Autodesk Inventor part; units mm, degrees
ref_plane "YZ Plane" through (0, 0, 0) normal (1, 0, 0) x (0, 1, 0)
ref_plane "XZ Plane" through (0, 0, 0) normal (0, 1, 0) x (-1, 0, 0)
ref_plane "XY Plane" through (0, 0, 0) normal (0, 0, 1) x (1, 0, 0)
sketch "Sketch1" plane through (0, 0, 0) normal (0, 0, 1) x (1, 0, 0)
  line L0 (0, 0) -> (25.4, 0)
  line L1 (25.4, 0) -> (25.4, 520.7)
  line L2 (25.4, 520.7) -> (0, 520.7)
  line L3 (0, 520.7) -> (0, 0)
  dimension "d0" = 25.4
  dimension "d1" = 520.7
extrude "Extrusion1" add sketch "Sketch1" along normal blind 25.4
shell "Shell1" thickness 3.175 removed faces 2 at (16.9333, 520.7, 8.4667) at (8.4667, 0, 8.4667)
sketch "Sketch2" plane through (0, 0, 0) normal (0, 0, -1) x (-1, 0, 0)
  line L0 (0, 520.7) -> (0, 0)
  line L1 (-25.4, 520.7) -> (0, 520.7)
  circle A0 centre (-12.7, 495.3) radius 3.175
  dimension "d5" = 12.7
  dimension "d6" = 25.4
  dimension "d7" = 6.35
extrude "Extrusion2" cut sketch "Sketch2" against normal through all
properties part number "CentralColumnInner" material "Aluminum-6061"
Read the model definition and answer for the solid it produces. Units are mm, in the model's axes. A direction names the side the tool comes from. Round coordinates to 2 decimals unless told otherwise and drop trailing zeros. Order: outer loops, then holes, each group sorted by start corner. A loop starts at its lowest first (then second) coordinate and runs counter-clockwise, first axis right, second up.
1) The part is cut by section A-A on z = 8.5. Write down the section's boundary in (x, y) (3 decimals), plus the area to 3 significant figures.
2) A flat-ended cylindrical pin translates along its axis: pin 1 (4 mm diameter, centred on x = 12.7, y = 495.3, fed in from +Z). Find the tip coordinate at first contact, or state that the pin passes through.
3) The part is cut by section B-B on y = 78. Write down the section's boundary in (x, z) (3 decimals).
4) The mould has two halves that part along Z. Classify faces 3 (the face through (13, 264, 0)), 4 (the face through (13, 264, 25.4)), 5 (the face through (13, 264, 3.175)), 6 (the face through (25.4, 257, 13)): released by +Z, released by -Z, zero draft, split by the parting line, or undercut.
5) Straight lines are drawn through the part: L1, parallel to X at y = 495.3, z = 24.75 (3 decimals); L2, parallel to Z at x = 4.5, y = 63 (3 decimals). For each, find the intervals that lie inside material, in ascending order.
6) For faces 1 (the face through (2, 520.7, 13)), 2 (the face through (13, 264, 22.225)), determine the directions among +Z, -Z, +X, -X, +Y, -Y from which every point of the face is accessible in a straight line to the end or side of a thin tool.
Resolved:
1. outline: (0, 0) - (3.175, 0) - (3.175, 520.7) - (0, 520.7) - close; (22.225, 0) - (25.4, 0) - (25.4, 520.7) - (22.225, 520.7) - close
1. area: 3,310 mm2
2. pin 1: passes through
3. outline: (0, 0) - (25.4, 0) - (25.4, 25.4) - (0, 25.4) - close; hole (3.175, 3.175) - (22.225, 3.175) - (22.225, 22.225) - (3.175, 22.225) - close
4. face 3: released by -Z
4. face 4: released by +Z
4. face 5: undercut
4. face 6: zero draft
5. L1: x = 0 to 9.525, 15.875 to 25.4
5. L2: z = 0 to 3.175, 22.225 to 25.4
6. face 1: +Z, -Z, +X, -X, +Y
6. face 2: +Y, -Y
